Verification items for this drawing (mm, ordinates from the low corner). A direction names the side the tool comes from. Give positions to 0.01 mm unless a question says otherwise; leave off trailing zeros. Loops run counter-clockwise (first coordinate to the right, second up) from the corner with the lowest first, then second, coordinate; pieces in that order, holes last. Notation, with made-up numbers: (2, -38.75) -> (9, -38.75) arc R22 cw to (9, -7.75) -> close; hole circle Ø10 at (54, 74.25). An arc over 180 degrees is marked (long way). Write each question's results on one line, items separated by ' | '. Start each with the question number.
1) Set-up check for the marked faces 1 and 2: record each of +Z, -Z, +X, -X, +Y, -Y from which the full face is reachable in a straight line by a thin tool's end or side.
2) Sectioned sample at B-B on z = 33.5. Record the cut outline in (x, y).
3) Sectioned sample at A-A on x = 45. Record the cut outline in (y, z), then the cut area to 4 significant figures.
4) Scan lines: line 1 (Y direction, x = 60, z = 3); line 2 (X direction, y = 30, z = 70.5); line 3 (Z direction, x = 63.5, y = 35.5). Record each from-to range of solid material in increasing order. Write a range as from..to.
5) Sectioned sample at C-C on z = 92. Record the cut outline in (x, y).
6) Depth check by flat-ended pin: pin 1 (4 mm diameter, centred on x = 30, y = 4.25, fed in from -Z); pin 2 (6.5 mm diameter, centred on x = 23.5, y = 19.25, fed in from +Z). Enter the tip coordinate at first touch or a pass-through.
7) Sectioned sample at D-D on x = 68. Record the cut outline in (y, z), then the cut area to 3 significant figures.
8) Draft check along Y on the marked faces 3, 4 and 5. Enter one of: pulls with the +Y half, pulls with the -Y half, needs draft (parallel to the pull), parting line crosses it, or undercut.
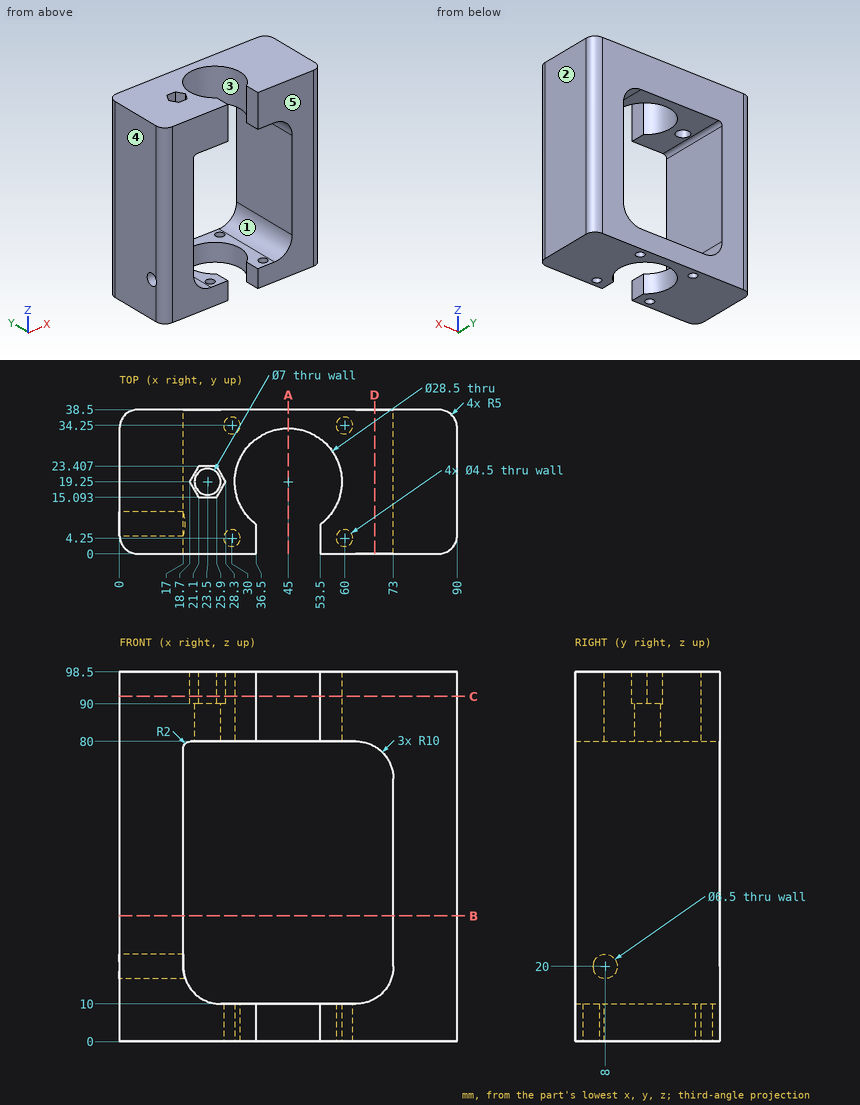
Result:
1) face 1: +Y, -Y | face 2: +Z, -Z, +X, +Y, -Y
2) outline: (0, 5) arc R5 ccw to (5, 0) -> (17, 0) -> (17, 38.5) -> (5, 38.5) arc R5 ccw to (0, 33.5) -> close; (73, 0) -> (85, 0) arc R5 ccw to (90, 5) -> (90, 33.5) arc R5 ccw to (85, 38.5) -> (73, 38.5) -> close
3) outline: (33.5, 0) -> (38.5, 0) -> (38.5, 10) -> (33.5, 10) -> close; (33.5, 80) -> (38.5, 80) -> (38.5, 98.5) -> (33.5, 98.5) -> close | area: 142.5 mm^2
4) line 1: 0..2, 6.5..32, 36.5..38.5 | line 2: 0..17, 72.99..90 | line 3: 0..10.01, 79.99..98.5
5) outline: (0, 5) arc R5 ccw to (5, 0) -> (36.5, 0) -> (36.5, 7.81) arc R14.25 cw (long way) to (53.5, 7.81) -> (53.5, 0) -> (85, 0) arc R5 ccw to (90, 5) -> (90, 33.5) arc R5 ccw to (85, 38.5) -> (5, 38.5) arc R5 ccw to (0, 33.5) -> close; hole (18.7, 19.25) -> (21.1, 15.09) -> (25.9, 15.09) -> (28.3, 19.25) -> (25.9, 23.41) -> (21.1, 23.41) -> close
6) pin 1: z = 80 | pin 2: z = 12.62
7) outline: (0, 0) -> (38.5, 0) -> (38.5, 11.34) -> (0, 11.34) -> close; (0, 78.66) -> (38.5, 78.66) -> (38.5, 98.5) -> (0, 98.5) -> close | area: 1,200 mm^2
8) face 3: undercut | face 4: needs draft | face 5: pulls with the -Y half
